Geometry check sheet. Reference: the model listing, model coordinates, mm. A direction names the side the tool comes from. Give positions to 0.01 mm unless a question says otherwise; leave off trailing zeros. Loops run counter-clockwise (first coordinate to the right, second up) from the corner with the lowest first, then second, coordinate; pieces in that order, holes last.
1. Release check for a two-part mould opening along X. For faces 1 (the cylindrical face through (0.08, 53.07, -51.74)), 2 (the cylindrical face through (-7.81, 35.12, -18.7)), 3 (the cylindrical face through (7.86, 35.09, -18.74)), 4 (the flat face through (-3.75, 7, 28)) record: +X half, -X half, draft (parallel to the pull), parting line (faces both ways), or undercut.
2. Cross-section at B-B, the plane z = 21. Record the cut outline in (x, y), plus the area to 4 significant figures.
3. Material ranges on L1, parallel to Y at x = -1.25, z = 9.5; L2, parallel to Y at x = 0, z = 8; L3, parallel to Y at x = 1.5, z = 23.5, recorded low to high.
4. Go/stop test with flat-tipped pins: pin 1 Ø0.8 at (x, z) = (0, 28.5) entering from +Y; pin 2 Ø3 at (x, y) = (-0.5, 3) entering from -Z; pin 3 Ø5 at (x, z) = (1.5, -21.5) entering from +Y. Record where each tip stops, or that it passes through.
5. Cross-section at A-A, the plane x = 0.5. Record the cut outline in (y, z) (3 decimals), plus the area to 3 significant figures.
6. Tool access check on faces 5 (the cylindrical face through (-7.81, 25.31, -24.05)), 6 (the flat face through (-0.053, 7.535, 8.91)), 7 (the flat face through (-6.25, 7, 19)), 8 (the flat face through (0, 2.5, 19)), 9 (the flat face through (0, 12.5, 29)). Record the directions out of +Z, -Z, +X, -X, +Y, -Y that give a thin tool (end or side, any length) a straight path to the whole face; none if there is none.
from build123d import *

# Parameters (mm, degrees)
BOSS_EXTRUDE1_DEPTH      = 8.75
BOSS_EXTRUDE1_DEPTH_BACK = 8.75
BOSS_EXTRUDE2_REACH      = 83.958
SKETCH2_W                = 2.5
SKETCH2_H                = 12.5
CUT_EXTRUDE1_START       = 2.5
SKETCH3_W                = 2.5
SKETCH3_H                = 22.5
CUT_EXTRUDE1_DEPTH       = 80.458449839
FILLET1_R                = 3.125


with BuildPart() as part:
    # Sketch1 → Boss-Extrude1 (new, two sides: drawn at the far end of the back side and taken through both)
    with BuildSketch(Plane(origin=(0, 0, 0), x_dir=(0, 0, -1), z_dir=(1, 0, 0)).offset(-BOSS_EXTRUDE1_DEPTH_BACK)):
        Polygon((-27.67766953, 2.5), (-27.67766953, 5), (-25.17766953, 5), (-27.67766953, 10), (-27.67766953, 12.5), (-30.17766953, 12.5), (-30.17766953, 0), (0, 0), (53.033008589, 53.033008589), (44.194173824, 61.871843354), (-5.17766953, 12.5), (-7.67766953, 12.5), (-7.67766953, 10), (-10.17766953, 5), (-7.67766953, 5), (-7.67766953, 2.5), align=None)
    extrude(amount=BOSS_EXTRUDE1_DEPTH + BOSS_EXTRUDE1_DEPTH_BACK)

    # Boss-Extrude2: up to this face of the body (flat: up to its plane)
    boss_extrude2_end = Plane(part.part.faces().sort_by_distance((0, 6.25, 30.17766953))[0])
    # Sketch2 → Boss-Extrude2 (add, up to the picked face)
    with BuildSketch(Plane.XY, mode=Mode.PRIVATE) as boss_extrude2_sk1:
        with Locations((-7.5, 6.25)):
            Rectangle(SKETCH2_W, SKETCH2_H)
    boss_extrude2_tool1 = split(extrude(boss_extrude2_sk1.sketch, amount=BOSS_EXTRUDE2_REACH, mode=Mode.PRIVATE), bisect_by=boss_extrude2_end, keep=Keep.BOTH, mode=Mode.PRIVATE)
    # Sketch2 → Boss-Extrude2 (add, up to the picked face)
    with BuildSketch(Plane.XY, mode=Mode.PRIVATE) as boss_extrude2_sk2:
        with Locations((7.5, 6.25)):
            Rectangle(SKETCH2_W, SKETCH2_H)
    boss_extrude2_tool2 = split(extrude(boss_extrude2_sk2.sketch, amount=BOSS_EXTRUDE2_REACH, mode=Mode.PRIVATE), bisect_by=boss_extrude2_end, keep=Keep.BOTH, mode=Mode.PRIVATE)
    add(boss_extrude2_tool1.solids().sort_by(Axis((-7.5, 6.25, 0), (0, 0, 1)))[0])
    add(boss_extrude2_tool2.solids().sort_by(Axis((7.5, 6.25, 0), (0, 0, 1)))[0])

    # Sketch3 → Cut-Extrude1 (cut, through all)
    with BuildSketch(Plane(origin=(0, 0, 0), x_dir=(1, 0, 0), z_dir=(0, 1, 0)).offset(CUT_EXTRUDE1_START)):
        with Locations((-5, -18.92766953)):
            Rectangle(SKETCH3_W, SKETCH3_H)
        with Locations((5, -18.92766953)):
            Rectangle(SKETCH3_W, SKETCH3_H)
    extrude(amount=CUT_EXTRUDE1_DEPTH, mode=Mode.SUBTRACT)

    # Fillet1
    fillet1_edges = [part.edges().sort_by_distance(p)[0] for p in [
        (0, 61.871843354, -44.194173824),
        (0, 53.033008589, -53.033008589),
        (-8.75, 26.516504294, -26.516504294),
        (-8.75, 57.452425971, -48.613591207),
        (-8.75, 37.185921677, -19.508252147),
        (8.75, 26.516504294, -26.516504294),
        (8.75, 57.452425971, -48.613591207),
        (8.75, 37.185921677, -19.508252147),
    ]]
    fillet(fillet1_edges, radius=FILLET1_R)


solid = part.part
Result:
1. face 1: draft
1. face 2: -X half
1. face 3: +X half
1. face 4: undercut
2. outline: (-8.75, 0) - (8.75, 0) - (8.75, 12.5) - (6.25, 12.5) - (6.25, 2.5) - (-6.25, 2.5) - (-6.25, 12.5) - (-8.75, 12.5) - close
2. area: 93.75 mm2
3. L1: y = 0 to 2.5, 5 to 6.36
3. L2: y = 0 to 2.5, 5 to 9.36
3. L3: y = 0 to 2.5
4. pin 1: stops at y = 12.5
4. pin 2: stops at z = -4.5
4. pin 3: stops at y = 41.68
5. outline: (0, 0) - (50.823, -50.823) arc R3.125 ccw to (55.243, -50.823) - (59.662, -46.404) arc R3.125 ccw to (59.662, -41.984) - (12.5, 5.178) - (12.5, 7.678) - (10, 7.678) - (5, 10.178) - (5, 7.678) - (2.5, 7.678) - (2.5, 27.678) - (5, 27.678) - (5, 25.178) - (10, 27.678) - (12.5, 27.678) - (12.5, 30.178) - (0, 30.178) - close
5. area: 1,060 mm2
6. face 5: -Z, -X, -Y
6. face 6: +Y
6. face 7: +Z, +Y
6. face 8: none
6. face 9: +Z, +X, -X, +Y
